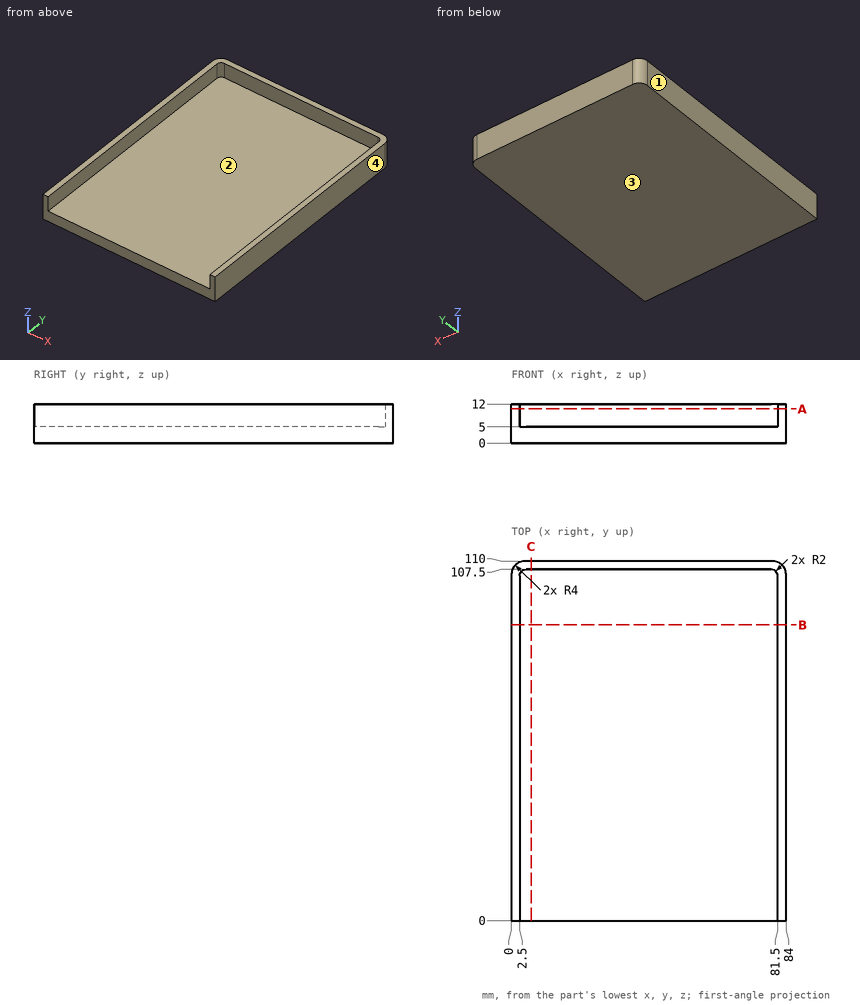
Study the drawing (mm; zero at the part's minimum x, y, z) and answer. Coordinates: 2 decimals unless noted, no trailing zeros. Loops run counter-clockwise (first coordinate to the right, second up) from the corner with the lowest first, then second, coordinate; pieces in that order, holes last. Notation, with made-up numbers: M 67,-38.5 L 125,-38.5 A6 cw 125,-33.5 Z; hole C 8.25,66.25 d1. An arc over 180 degrees is marked long. Answer in a Markdown table with one row per item.
1) Find section A-A (z = 10.5). Determine the outline of the cut face in (x, y), then the cut area to 3 significant figures.
Answers below:
| item | result |
|---|---|
| outline | M 0,0 L 2.5,0 L 2.5,105.5 A2 cw 4.5,107.5 L 79.5,107.5 A2 cw 81.5,105.5 L 81.5,0 L 84,0 L 84,106 A4 ccw 80,110 L 4,110 A4 ccw 0,106 Z |
| area | 742 mm^2 |
2) Find the intervals of material crossed by probe 1 along X at (y, z) = (64.5, 7.5); probe 2 along Z at (x, y) = (65, 69); probe 3 along Y at (x, z) = (63.5, 9), in increasing order.
Answers below:
| item | result |
|---|---|
| probe 1 | 0 to 2.5, 81.5 to 84 |
| probe 2 | 0 to 5 |
| probe 3 | 107.5 to 110 |
3) Find section B-B (y = 90.5). Determine the outline of the cut face in (x, z).
Answers below:
| item | result |
|---|---|
| outline | M 0,0 L 84,0 L 84,12 L 81.5,12 L 81.5,5 L 2.5,5 L 2.5,12 L 0,12 Z |
4) Determine the mould class of the marked faces 1, 2, 3 and 4 for opening direction X: released by +X, released by -X, zero draft, split by the parting line, or undercut.
Answers below:
| item | result |
|---|---|
| face 1 | released by -X |
| face 2 | undercut |
| face 3 | zero draft |
| face 4 | released by +X |
5) Given pin 1 (3 mm diameter, centred on x = 58, z = 7, fed in from -Y); pin 2 (4 mm diameter, centred on x = 54.5, y = 67.5, fed in from +Z), each flat-ended and moving along its own axis, determine where each tip first touches the part or whether it passes through.
Answers below:
| item | result |
|---|---|
| pin 1 | y = 107.5 |
| pin 2 | z = 5 |
6) Find section C-C (x = 6). Determine the outline of the cut face in (y, z).
Answers below:
| item | result |
|---|---|
| outline | M 0,0 L 110,0 L 110,12 L 107.5,12 L 107.5,5 L 0,5 Z |
